from build123d import *

# Parameters (mm, degrees)
F1_DEPTH = 163
F2_R     = 2
F3_R     = 1
F4_R     = 1


with BuildPart() as f1:
    # F0 (on Front) → F1 (new body)
    with BuildSketch(Plane.XZ):
        Polygon((8.75, 0), (0, 0), (0, -2), (6.75, -2), (6.75, -4.25), (6.25, -4.25), (6.25, -5.75), (8.75, -5.75), align=None)
    extrude(amount=F1_DEPTH)

    # F2
    f2_edges = [f1.edges().sort_by_distance(p)[0] for p in [
        (8.75, -81.5, 0),
    ]]
    fillet(f2_edges, radius=F2_R)

    # F3
    f3_edges = [f1.edges().sort_by_distance(p)[0] for p in [
        (6.75, -81.5, -2),
    ]]
    fillet(f3_edges, radius=F3_R)

    # F4
    f4_edges = [f1.edges().sort_by_distance(p)[0] for p in [
        (8.75, -81.5, -5.75),
    ]]
    fillet(f4_edges, radius=F4_R)

    # F5: F1 across plane


with BuildPart() as f1_1:
    add(f1.part)
    add(f1.part.mirror(Plane.YZ))


solid = f1_1.part
Source: CAD feature listing. Evaluate the final solid. Frame: model axes, mm. A direction names the side the tool comes from. Give positions to 0.01 mm unless a question says otherwise; leave off trailing zeros. Write each loop counter-clockwise with the first axis right and the second up, starting at its lowest first coordinate (ties: lowest second). Pieces come first, ordered by that corner, then holes. Notation, with made-up numbers: M 20.25,62.5 L 52.25,62.5 A14 cw 52.25,82.5 Z; hole C 76,86.25 d5. An arc over 180 degrees is marked long. Return JSON: item names as keys, results as strings. Group by question number.
1) Cut plane A-A, the plane y = -43. Output: boundary loops of the cut face in (x, z).
2) Ray query, L1, parallel to X at y = -39, z = -3.1; L2, parallel to Z at x = 0.5, y = -17. Return the intervals inside material, ascending.
3) Set-up query: faces 1 (the face through (0, -80, 0)), 2 (the face through (0, -80, -2)). Return all of +Z, -Z, +X, -X, +Y, -Y with unobstructed straight access to the full face (end or side cutting, diameter ignored); none if empty.
4) Cut plane B-B, the plane x = 1.5. Output: boundary loops of the cut face in (y, z), then the cut area to 3 significant figures.
5) First-contact query: pin 1 Ø1.5 at (x, y) = (-1, -56) entering from -Z. Flat tip, straight axial feed; report the tip coordinate or a pass-through.
6) Cut plane C-C, the plane z = -0.9. Output: boundary loops of the cut face in (x, y), then the cut area to 3 significant figures.
Data:
{
 "1": {"outline": "M -8.75,-4.75 A1 ccw -7.75,-5.75 L -6.25,-5.75 L -6.25,-4.25 L -6.75,-4.25 L -6.75,-3 A1 cw -5.75,-2 L 5.75,-2 A1 cw 6.75,-3 L 6.75,-4.25 L 6.25,-4.25 L 6.25,-5.75 L 7.75,-5.75 A1 ccw 8.75,-4.75 L 8.75,-2 A2 ccw 6.75,0 L -6.75,0 A2 ccw -8.75,-2 Z"},
 "2": {"L1": "x = -8.75 to -6.75, 6.75 to 8.75", "L2": "z = -2 to 0"},
 "3": {"face 1": "+Z, +X, -X, +Y, -Y", "face 2": "-Z, +Y, -Y"},
 "4": {"outline": "M -163,-2 L 0,-2 L 0,0 L -163,0 Z", "area": "326 mm²"},
 "5": {"pin 1": "stops at z = -2"},
 "6": {"outline": "M -8.42,-163 L 8.42,-163 L 8.42,0 L -8.42,0 Z", "area": "2,750 mm²"}
}
